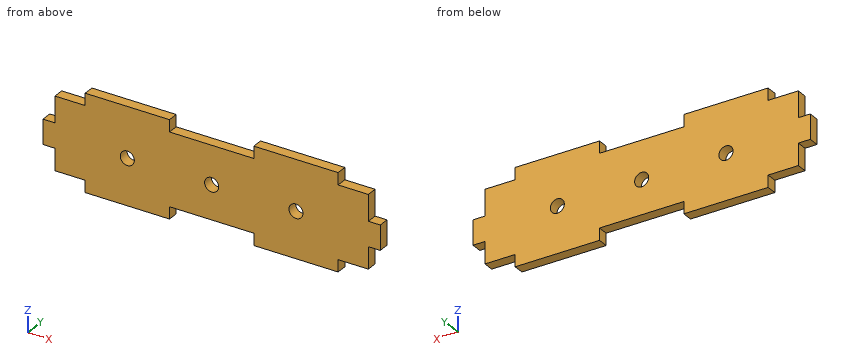
```python
from build123d import *

# Parameters (mm, degrees)
F1_DEPTH = 19.05
F2_R     = 12.7
F3_DEPTH = 19.051


with BuildPart() as f1:
    # F0 (on Front) → F1 (new body)
    with BuildSketch(Plane.XZ):
        Polygon((-86.786535, 62.306761), (-86.786535, 17.856761), (-65.196535, 17.856761), (-65.196535, -21.513239), (-10.586535, -21.513239), (-10.586535, -43.103239), (141.813465, -43.103239), (141.813465, -21.513239), (294.213465, -21.513239), (294.213465, -43.103239), (446.613465, -43.103239), (446.613465, -21.513239), (501.223465, -21.513239), (501.223465, 17.856761), (522.813465, 17.856761), (522.813465, 62.306761), (501.223465, 62.306761), (501.223465, 109.296761), (446.613465, 109.296761), (446.613465, 130.886761), (294.213465, 130.886761), (294.213465, 109.296761), (141.813465, 109.296761), (141.813465, 130.886761), (-10.586535, 130.886761), (-10.586535, 109.296761), (-65.196535, 109.296761), (-65.196535, 62.306761), align=None)
    extrude(amount=F1_DEPTH)

    # F2 (on face) → F3 (cut, through all)
    with BuildSketch(Plane.XZ.offset(19.05)):
        with Locations((65.613465, 40.081761)):
            Circle(F2_R)
        with Locations((218.013465, 40.081761)):
            Circle(F2_R)
        with Locations((370.413465, 40.081761)):
            Circle(F2_R)
    extrude(amount=-F3_DEPTH, mode=Mode.SUBTRACT)


solid = f1.part
```
Verification items for the finished model (mm, model axes). Round coordinates to 2 decimals unless told otherwise and drop trailing zeros. Write each loop counter-clockwise with the first axis right and the second up, starting at its lowest first coordinate (ties: lowest second). Pieces come first, ordered by that corner, then holes. Notation, with made-up numbers: (73, -20) -> (111, -20) arc R14 cw to (111, -3) -> close; hole circle Ø9 at (11.25, 3). An arc over 180 degrees is marked (long way). Write each question's results on one line, items separated by ' | '.
Q1. Go/stop test with flat-tipped pins: pin 1 Ø5.5 at (y, z) = (-7, 4) entering from +X; pin 2 Ø4 at (y, z) = (-2.5, 111) entering from -X; pin 3 Ø5.5 at (y, z) = (-11.5, -35) entering from +X; pin 4 Ø15 at (x, z) = (370.41, 40.08) entering from -Y. Record where each tip stops, or that it passes through.
Derived:
pin 1: stops at x = 501.22 | pin 2: stops at x = -65.2 | pin 3: stops at x = 446.61 | pin 4: passes through
Q2. Sectioned sample at A-A, the plane z = 46. Record the boundary of the cut face in (x, y).
Derived:
outline: (-86.79, -19.05) -> (54.38, -19.05) -> (54.38, 0) -> (-86.79, 0) -> close; (76.85, -19.05) -> (206.78, -19.05) -> (206.78, 0) -> (76.85, 0) -> close; (229.25, -19.05) -> (359.18, -19.05) -> (359.18, 0) -> (229.25, 0) -> close; (381.65, -19.05) -> (522.81, -19.05) -> (522.81, 0) -> (381.65, 0) -> close
Q3. Sectioned sample at B-B, the plane y = -5.5. Give the number of separate pieces and of enclosed holes in the cut face, and give its area (3 significant figures).
Derived:
separate pieces: 1 | enclosed holes: 3 | area: 87,700 mm²
Q4. Sectioned sample at C-C, the plane x = 65. Record the boundary of the cut face in (y, z), and give its area (3 significant figures).
Derived:
outline: (-19.05, -43.1) -> (0, -43.1) -> (0, 27.4) -> (-19.05, 27.4) -> close; (-19.05, 52.77) -> (0, 52.77) -> (0, 130.89) -> (-19.05, 130.89) -> close | area: 2,830 mm²
Q5. Thickness scan on probe 1 along X at (y, z) = (-3.25, -30); probe 2 along X at (y, z) = (-9.75, 37); probe 3 along X at (y, z) = (-13.75, 90). Record the ranges inside material, lowest first.
Derived:
probe 1: x = -10.59 to 141.81, 294.21 to 446.61 | probe 2: x = -86.79 to 53.29, 77.93 to 205.69, 230.33 to 358.09, 382.73 to 522.81 | probe 3: x = -65.2 to 501.22
Q6. Sectioned sample at D-D, the plane z = 74. Record the boundary of the cut face in (x, y), and give its area (3 significant figures).
Derived:
outline: (-65.2, -19.05) -> (501.22, -19.05) -> (501.22, 0) -> (-65.2, 0) -> close | area: 10,800 mm²
